```python
from build123d import *

# Parameters (mm, degrees)
SKETCH_1_R          = 10
EXTRUDE_1_DEPTH     = 18
CUT_EXTRUDE_1_DEPTH = 18
SKETCH_3_R          = 4
CUT_EXTRUDE_2_DEPTH = 18


with BuildPart() as part:
    # 스케치1 → 보스-돌출1 (new body)
    with BuildSketch(Plane.XY):
        Circle(SKETCH_1_R)
    extrude(amount=EXTRUDE_1_DEPTH)

    # 스케치2 → 컷-돌출1 (cut)
    with BuildSketch(Plane.XY.offset(18)):
        with BuildLine():
            Line((-1.271266061, 9.918864986), (-0.440085126, 9.489416934))
            Line((-0.440085126, 9.489416934), (0, 10))
            ThreePointArc((0, 10), (-0.652192749, 10.218898871), (-1.271266061, 9.918864986))
        make_face()
        with BuildLine():
            Line((0.52024544, 9.986458065), (1.261388044, 9.415498333))
            Line((1.261388044, 9.415498333), (1.785568948, 9.839295886))
            ThreePointArc((1.785568948, 9.839295886), (1.182943108, 10.171130474), (0.52024544, 9.986458065))
        make_face()
        with BuildLine():
            Line((2.295035824, 9.733078165), (2.922319165, 9.038957869))
            Line((2.922319165, 9.038957869), (3.513748241, 9.362348706))
            ThreePointArc((3.513748241, 9.362348706), (2.980058199, 9.796453575), (2.295035824, 9.733078165))
        make_face()
        with BuildLine():
            Line((3.996061868, 9.166869125), (4.489324543, 8.371897862))
            Line((4.489324543, 8.371897862), (5.128992774, 8.584487936))
            ThreePointArc((5.128992774, 8.584487936), (4.681391768, 9.106910598), (3.996061868, 9.166869125))
        make_face()
        with BuildLine():
            Line((5.568651195, 8.306029368), (5.912039336, 7.435758169))
            Line((5.912039336, 7.435758169), (6.579387259, 7.53071466))
            ThreePointArc((6.579387259, 7.53071466), (6.232261554, 8.12466402), (5.568651195, 8.306029368))
        make_face()
        with BuildLine():
            Line((6.962259492, 7.178226993), (7.144736321, 6.26062709))
            Line((7.144736321, 6.26062709), (7.818314825, 6.234898019))
            ThreePointArc((7.818314825, 6.234898019), (7.582821326, 6.881284056), (6.962259492, 7.178226993))
        make_face()
        with BuildLine():
            Line((8.13209504, 5.819710497), (8.147795602, 4.884274306))
            Line((8.147795602, 4.884274306), (8.805955319, 4.738686625))
            ThreePointArc((8.805955319, 4.738686625), (8.689662981, 5.416733961), (8.13209504, 5.819710497))
        make_face()
        with BuildLine():
            Line((9.040558362, 4.274143716), (8.888978028, 3.350936926))
            Line((8.888978028, 3.350936926), (9.510565163, 3.090169944))
            ThreePointArc((9.510565163, 3.090169944), (9.517211718, 3.778085579), (9.040558362, 4.274143716))
        make_face()
        with BuildLine():
            Line((9.658450699, 2.59120244), (9.344461386, 1.709897677))
            Line((9.344461386, 1.709897677), (9.909497618, 1.342332658))
            ThreePointArc((9.909497618, 1.342332658), (10.038869439, 2.018006418), (9.658450699, 2.59120244))
        make_face()
        with BuildLine():
            Line((9.965912485, 0.824977785), (9.499606067, 0.013900909))
            Line((9.499606067, 0.013900909), (9.989930665, -0.448648304))
            ThreePointArc((9.989930665, -0.448648304), (10.237869637, 0.19306687), (9.965912485, 0.824977785))
        make_face()
        with BuildLine():
            Line((9.953061643, -0.967762334), (9.349425592, -1.682542646))
            Line((9.349425592, -1.682542646), (9.749279122, -2.22520934))
            ThreePointArc((9.749279122, -2.22520934), (10.107816281, -1.638078006), (9.953061643, -0.967762334))
        make_face()
        with BuildLine():
            Line((9.62031121, -2.729397776), (8.898746887, -3.324907895))
            Line((8.898746887, -3.324907895), (9.195277726, -3.930250317))
            ThreePointArc((9.195277726, -3.930250317), (9.652889393, -3.416573707), (9.62031121, -2.729397776))
        make_face()
        with BuildLine():
            Line((8.97835606, -4.403308127), (8.162055134, -4.860407869))
            Line((8.162055134, -4.860407869), (8.345732537, -5.508969815))
            ThreePointArc((8.345732537, -5.508969815), (8.887710697, -5.085257917), (8.97835606, -4.403308127))
        make_face()
        with BuildLine():
            Line((8.047829158, -5.935692533), (7.163028213, -6.239690335))
            Line((7.163028213, -6.239690335), (7.227948638, -6.91062649))
            ThreePointArc((7.227948638, -6.91062649), (7.836873667, -6.590497754), (8.047829158, -5.935692533))
        make_face()
        with BuildLine():
            Line((6.858638405, -7.277298896), (5.933775673, -7.418424019))
            Line((5.933775673, -7.418424019), (5.877852523, -8.090169944))
            ThreePointArc((5.877852523, -8.090169944), (6.534153069, -7.883913571), (6.858638405, -7.277298896))
        make_face()
        with BuildLine():
            Line((5.449005371, -8.385006885), (4.513806699, -8.358723452))
            Line((4.513806699, -8.358723452), (4.338837391, -9.009688679))
            ThreePointArc((4.338837391, -9.009688679), (5.021419415, -8.923933919), (5.449005371, -8.385006885))
        make_face()
        with BuildLine():
            Line((3.864236821, -9.223213854), (2.948760264, -9.030366635))
            Line((2.948760264, -9.030366635), (2.660368456, -9.639628607))
            ThreePointArc((2.660368456, -9.639628607), (3.347293209, -9.677131687), (3.864236821, -9.223213854))
        make_face()
        with BuildLine():
            Line((2.15526852, -9.76497914), (1.288938249, -9.411766404))
            Line((1.288938249, -9.411766404), (0.896393089, -9.95974294))
            ThreePointArc((0.896393089, -9.95974294), (1.565582245, -10.119298481), (2.15526852, -9.76497914))
        make_face()
        with BuildLine():
            Line((0.377028115, -9.992889962), (-0.412311303, -9.490664258))
            Line((-0.412311303, -9.490664258), (-0.896393089, -9.95974294))
            ThreePointArc((-0.896393089, -9.95974294), (-0.26644782, -10.236222696), (0.377028115, -9.992889962))
        make_face()
        with BuildLine():
            Line((-1.413330284, -9.899621079), (-2.10030883, -9.264524353))
            Line((-2.10030883, -9.264524353), (-2.660368456, -9.639628607))
            ThreePointArc((-2.660368456, -9.639628607), (-2.089914033, -10.024146291), (-1.413330284, -9.899621079))
        make_face()
        with BuildLine():
            Line((-3.158263084, -9.488170229), (-3.720800703, -8.740615012))
            Line((-3.720800703, -8.740615012), (-4.338837391, -9.009688679))
            ThreePointArc((-4.338837391, -9.009688679), (-3.846208689, -9.489885576), (-3.158263084, -9.488170229))
        make_face()
        with BuildLine():
            Line((-4.801686711, -8.77176178), (-5.221702981, -7.935775113))
            Line((-5.221702981, -7.935775113), (-5.877852523, -8.090169944))
            ThreePointArc((-5.877852523, -8.090169944), (-5.478883034, -8.65061213), (-4.801686711, -8.77176178))
        make_face()
        with BuildLine():
            Line((-6.290780175, -7.773421691), (-6.554775427, -6.875872872))
            Line((-6.554775427, -6.875872872), (-7.227948638, -6.91062649))
            ThreePointArc((-7.227948638, -6.91062649), (-6.935461569, -7.533300893), (-6.290780175, -7.773421691))
        make_face()
        with BuildLine():
            Line((-7.577682789, -6.525237433), (-7.677171999, -5.59497442))
            Line((-7.677171999, -5.59497442), (-8.345732537, -5.508969815))
            ThreePointArc((-8.345732537, -5.508969815), (-8.169128664, -6.173863166), (-7.577682789, -6.525237433))
        make_face()
        with BuildLine():
            Line((-8.621032443, -5.067326674), (-8.552817945, -4.134248887))
            Line((-8.552817945, -4.134248887), (-9.195277726, -3.930250317))
            ThreePointArc((-9.195277726, -3.930250317), (-9.140233241, -4.615992398), (-8.621032443, -5.067326674))
        make_face()
        with BuildLine():
            Line((-9.387295021, -3.446547867), (-9.153569286, -2.540645192))
            Line((-9.153569286, -2.540645192), (-9.749279122, -2.22520934))
            ThreePointArc((-9.749279122, -2.22520934), (-9.817563202, -2.909759836), (-9.387295021, -3.446547867))
        make_face()
        with BuildLine():
            Line((-9.851842212, -1.714994175), (-9.460117378, -0.865383071))
            Line((-9.460117378, -0.865383071), (-9.989930665, -0.448648304))
            ThreePointArc((-9.989930665, -0.448648304), (-10.179348603, -1.110005198), (-9.851842212, -1.714994175))
        make_face()
        with BuildLine():
            Line((-9.99974309, 0.07168084), (-9.462609514, 0.837693175))
            Line((-9.462609514, 0.837693175), (-9.909497618, 1.342332658))
            ThreePointArc((-9.909497618, 1.342332658), (-10.213961365, 0.725425919), (-9.99974309, 0.07168084))
        make_face()
        with BuildLine():
            Line((-9.826243996, 1.856051975), (-9.160965594, 2.513845272))
            Line((-9.160965594, 2.513845272), (-9.510565163, 3.090169944))
            ThreePointArc((-9.510565163, 3.090169944), (-9.920289004, 2.537541251), (-9.826243996, 1.856051975))
        make_face()
        with BuildLine():
            Line((-9.336921335, 3.580768071), (-8.564880702, 4.109200314))
            Line((-8.564880702, 4.109200314), (-8.805955319, 4.738686625))
            ThreePointArc((-8.805955319, 4.738686625), (-9.307770392, 4.268097919), (-9.336921335, 3.580768071))
        make_face()
        with BuildLine():
            Line((-8.54750234, 5.190395336), (-7.693513497, 5.572482277))
            Line((-7.693513497, 5.572482277), (-7.818314825, 6.234898019))
            ThreePointArc((-7.818314825, 6.234898019), (-8.396092381, 5.861474409), (-8.54750234, 5.190395336))
        make_face()
        with BuildLine():
            Line((-7.483359587, 6.633199024), (-6.574870438, 6.856660075))
            Line((-6.574870438, 6.856660075), (-6.579387259, 7.53071466))
            ThreePointArc((-6.579387259, 7.53071466), (-7.214557053, 7.266458288), (-7.483359587, 6.633199024))
        make_face()
        with BuildLine():
            Line((-6.1786955, 7.862806237), (-5.244905634, 7.920459176))
            Line((-5.244905634, 7.920459176), (-5.128992774, 8.584487936))
            ThreePointArc((-5.128992774, 8.584487936), (-5.801139925, 8.437892218), (-6.1786955, 7.862806237))
        make_face()
        with BuildLine():
            Line((-4.675443055, 8.839696388), (-3.746365247, 8.729688202))
            Line((-3.746365247, 8.729688202), (-3.513748241, 9.362348706))
            ThreePointArc((-3.513748241, 9.362348706), (-4.201269387, 9.33812535), (-4.675443055, 8.839696388))
        make_face()
        with BuildLine():
            Line((-3.021918024, 9.532471424), (-2.127413598, 9.258337866))
            Line((-2.127413598, 9.258337866), (-1.785568948, 9.839295886))
            ThreePointArc((-1.785568948, 9.839295886), (-2.466366594, 9.93822345), (-3.021918024, 9.532471424))
        make_face()
    extrude(amount=-CUT_EXTRUDE_1_DEPTH, mode=Mode.SUBTRACT)

    # 스케치3 → 컷-돌출2 (cut)
    with BuildSketch(Plane.XY.offset(18)):
        Circle(SKETCH_3_R)
    extrude(amount=-CUT_EXTRUDE_2_DEPTH, mode=Mode.SUBTRACT)


solid = part.part
```
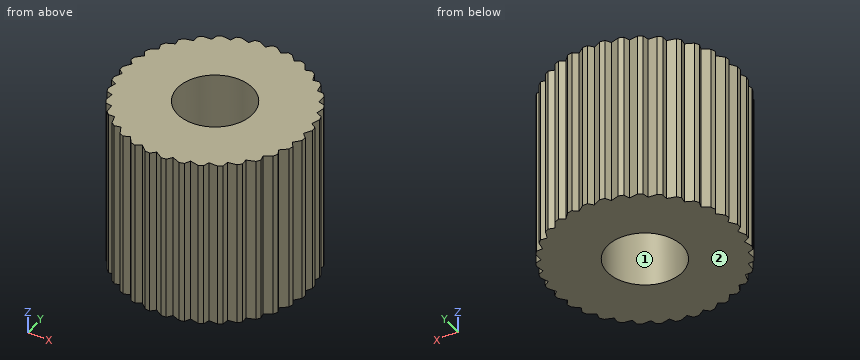
The model under review builds one solid part; all positions refer to its coordinate system, in mm. Face numbers are marked on the shaded views. Give positions to 0.01 mm unless a question says otherwise; leave off trailing zeros. Answer in a Markdown table with one row per item. Add a question column.
1. Wall thickness on line 1 along X through (y, z) = (2, 12.5); line 2 along X through (y, z) = (-1.5, 16.75); line 3 along Y through (x, z) = (0.5, 7): over which ranges is each line inside the solid? List them lowest first. Write a range as [from, to].
2. Draft analysis for pull direction Y (two halves, no side actions). For the marked faces 1 and 2, state which applies: +Y half, -Y half, draft (parallel to the pull), parting line (faces both ways), or undercut.
3. Insertion check: P1, Ø3, axis at y = -6.5, z = 11.5, coming from the +X side; P2, Ø8, axis at x = 5.5, z = 16, coming from the -Y side (3 decimals); P3, Ø1, axis at y = -8, z = 5.5, coming from the -X side. Each pin has a flat end and moves straight along its axis. Give the tip position at first contact, or say it passes through.
Ans:
| question | item | result |
|---|---|---|
| 1 | line 1 | x = [-9.68, -3.46], [3.46, 9.45] |
| 1 | line 2 | x = [-9.75, -3.71], [3.71, 9.5] |
| 1 | line 3 | y = [-9.99, -3.97], [3.97, 9.99] |
| 2 | face 1 | undercut |
| 2 | face 2 | draft |
| 3 | P1 | stops at x = 8.35 |
| 3 | P2 | stops at y = -9.765 |
| 3 | P3 | stops at x = -6.37 |
